Part model, mm, in its own coordinate system. Give positions to 0.01 mm unless a question says otherwise; leave off trailing zeros. Order: outer loops, then holes, each group sorted by start corner. A loop starts at its lowest first (then second) coordinate and runs counter-clockwise, first axis right, second up. Notation, with made-up numbers: (-3, -2) -> (16, -2) arc R11 cw to (16, 8) -> close; hole circle Ø4 at (42, -36). An arc over 180 degrees is marked (long way). Write item = value, one per line. Start each with the question number.
Item 1: Band-saw the part on B-B on x = 0.5. Write the cut outline in (y, z) (3 decimals).
Item 2: Flat gauge pins, fed straight in: P1, Ø4, axis at x = 0, z = -9.525, coming from the -Y side; P2, Ø2, axis at x = 7.5, z = -3, coming from the +Y side. Where does each tip first touch, or does it go through?
Item 3: Pull direction Z, two halves, no side cores. Call faces 1 (the face through (0, -6, -15.875)), 2 (the face through (-0.688, -6.261, -12.624)), 3 (the face through (0, -12.7, -13)): +Z half, -Z half, draft (parallel to the pull), parting line (faces both ways), or undercut.
Item 4: Band-saw the part on A-A on y = -6.75. Write the cut outline in (x, z) (3 decimals).
Item 5: Drill centre lines: line 1 along Z through (x, y) = (0, -2.5) (3 decimals); line 2 along Z through (x, y) = (1, -6) (3 decimals); line 3 along Z through (x, y) = (1.5, -9) (3 decimals). Where is each one in solid material? Low to high.
Item 6: Band-saw the part on D-D on z = -9. Write the cut outline in (x, y) (3 decimals).
Item 7: Band-saw the part on C-C on y = -2.75. Write the cut outline in (x, z) (3 decimals), plus the area to 4 significant figures.
```python
from build123d import *

# Parameters (mm, degrees)
F0_W     = 19.05
F0_H     = 31.75
F0_R     = 3.175
F1_DEPTH = 12.7
F2_R     = 6.35
F3_DEPTH = 19.051


with BuildPart() as f1:
    # F0 (on Front) → F1 (new body)
    with BuildSketch(Plane.XZ):
        Rectangle(F0_W, F0_H)
        with Locations((0, -9.525)):
            Circle(F0_R, mode=Mode.SUBTRACT)
        with Locations((0, 9.525)):
            Circle(F0_R, mode=Mode.SUBTRACT)
    extrude(amount=F1_DEPTH)

    # F2 (on face) → F3 (cut, through all)
    with BuildSketch(Plane.YZ.offset(9.525)):
        with Locations((-12.7, 0)):
            Circle(F2_R)
    extrude(amount=-F3_DEPTH, mode=Mode.SUBTRACT)


solid = f1.part
```
Values found:
q1.outline = (-12.7, -15.875) -> (0, -15.875) -> (0, -12.66) -> (-12.7, -12.66) -> close; (-12.7, -6.39) -> (0, -6.39) -> (0, 6.39) -> (-12.7, 6.39) -> (-12.7, 6.35) arc R6.35 cw to (-12.7, -6.35) -> close; (-12.7, 12.66) -> (0, 12.66) -> (0, 15.875) -> (-12.7, 15.875) -> close
q2.P1 = through
q2.P2 = 0
q3.face_1 = -Z half
q3.face_2 = undercut
q3.face_3 = draft
q4.outline = (-9.525, -15.875) -> (9.525, -15.875) -> (9.525, -2.218) -> (-9.525, -2.218) -> close; (-9.525, 2.218) -> (9.525, 2.218) -> (9.525, 15.875) -> (-9.525, 15.875) -> close; hole circle Ø6.35 at (0, -9.525); hole circle Ø6.35 at (0, 9.525)
q5.line_1 = -15.875 to -12.7, -6.35 to 6.35, 12.7 to 15.875
q5.line_2 = -15.875 to -12.538, -6.512 to 6.512, 12.538 to 15.875
q5.line_3 = -15.875 to -12.323, -6.727 to -5.161, 5.161 to 6.727, 12.323 to 15.875
q6.outline = (-9.525, -12.7) -> (-3.131, -12.7) -> (-3.131, 0) -> (-9.525, 0) -> close; (3.131, -12.7) -> (9.525, -12.7) -> (9.525, 0) -> (3.131, 0) -> close
q7.outline = (-9.525, -15.875) -> (9.525, -15.875) -> (9.525, 15.875) -> (-9.525, 15.875) -> close; hole circle Ø6.35 at (0, -9.525); hole circle Ø6.35 at (0, 9.525)
q7.area = 541.5 mm^2
